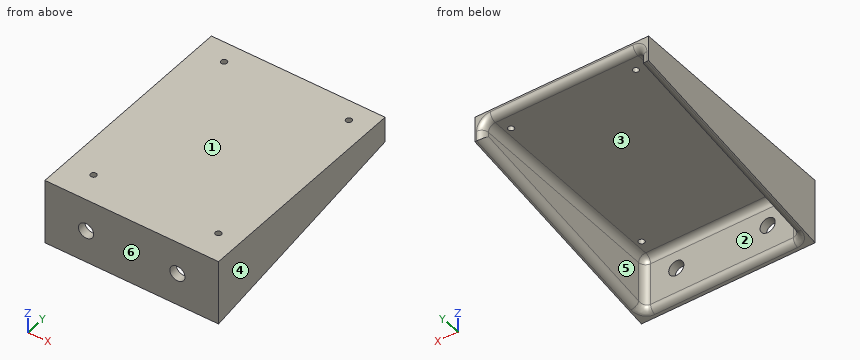
```python
from build123d import *

# Parameters (mm, degrees)
BOSS_EXTRUDE1_DEPTH        = 32.1564
SKETCH2_W                  = 57.9628
SKETCH2_H                  = 20.955
CUT_EXTRUDE1_DEPTH         = 80.772
M2_CLEARANCE_HOLE1_D       = 2.2
F_2_0_221_DIAMETER_HOLE1_D = 5.6134
FILLET1_R                  = 2.54


with BuildPart() as part:
    # Sketch1 → Boss-Extrude1 (new body, symmetric)
    with BuildSketch(Plane(origin=(0, 0, 0), x_dir=(0, 0, -1), z_dir=(1, 0, 0))):
        Polygon((0, 0), (24.13, 0), (9.4742, 83.947), (0, 83.947), align=None)
    extrude(amount=BOSS_EXTRUDE1_DEPTH, both=True)

    # Sketch2 → Cut-Extrude1 (cut)
    with BuildSketch(Plane(origin=(0, 83.947, 0), x_dir=(1, 0, 0), z_dir=(0, 1, 0))):
        with Locations((0, 13.6525)):
            Rectangle(SKETCH2_W, SKETCH2_H)
    extrude(amount=-CUT_EXTRUDE1_DEPTH, mode=Mode.SUBTRACT)

    # M2 Clearance Hole1 (through all)
    with Locations(Plane.XY):
        with Locations((-21.971, 76.454), (24.257, 76.454), (24.257, 10.668), (-21.971, 10.668)):
            Hole(M2_CLEARANCE_HOLE1_D / 2)

    # #2 (0.221) Diameter Hole1 (through all)
    with Locations(Plane(origin=(0, 0, 0), x_dir=(-1, 0, 0), z_dir=(0, -1, 0))):
        with Locations((-16.9164, 12.065), (16.9164, 12.065)):
            Hole(F_2_0_221_DIAMETER_HOLE1_D / 2)

    # Fillet1
    fillet1_edges = [part.edges().sort_by_distance(p)[0] for p in [
        (0, 3.175, -23.575695915),
        (28.9814, 43.561, -16.524947958),
        (-28.9814, 43.561, -16.524947958),
        (-28.9814, 43.561, -3.175),
        (-28.9814, 83.947, -6.3246),
        (0, 83.947, -3.175),
        (28.9814, 83.947, -6.3246),
        (28.9814, 3.175, -13.375347958),
        (0, 3.175, -3.175),
        (-28.9814, 3.175, -13.375347958),
        (28.9814, 43.561, -3.175),
    ]]
    fillet(fillet1_edges, radius=FILLET1_R)


solid = part.part
```
Part model, mm, in its own coordinate system. Face numbers are marked on the shaded views. A direction names the side the tool comes from. Coordinates: 2 decimals unless noted, no trailing zeros. Order: outer loops, then holes, each group sorted by start corner. A loop starts at its lowest first (then second) coordinate and runs counter-clockwise, first axis right, second up. Notation, with made-up numbers: (4.25, 86.5) -> (27.25, 86.5) arc R6 ccw to (27.25, 95.5) -> close; hole circle Ø10 at (36.5, 58). An arc over 180 degrees is marked (long way). Put each result on its own line as item: value. Start each with the question number.
(1) Band-saw the part on A-A (x = -7.5). Give the cut face in (y, z) (3 decimals).
(2) Probe line 1 along X through (y, z) = (8.5, -19.75); line 2 along Y through (x, z) = (-6.5, -8) (3 decimals); line 3 along Z through (x, y) = (23, 30) (3 decimals). List the from-to ranges inside material, lowest first. Write a range as [from, to].
(3) Pin check, flat tips, straight feed: pin 1 Ø4 at (x, y) = (-25.5, 17.5) entering from -Z; pin 2 Ø3.5 at (x, y) = (-21.971, 76.454) entering from -Z (3 decimals); pin 3 Ø6.5 at (x, z) = (16.92, -12.06) entering from +Y (3 decimals); pin 4 Ø1.3 at (x, y) = (24.257, 76.454) entering from -Z. Stop position of each tip, or through.
(4) Mould opens along X. For the marked faces 1, 2, 3 and 4 say: pulls with the +X half, pulls with the -X half, needs draft (parallel to the pull), parting line crosses it, or undercut.
(5) Which spindle directions (+Z, -Z, +X, -X, +Y, -Y) get a long thin tool onto all of the face, cutting with end or side? Do the marked faces 5 and 6. Say none if no direction does.
Determined:
1. outline: (0, -24.13) -> (1.072, -23.943) arc R2.54 ccw to (3.175, -21.441) -> (3.175, -5.715) arc R2.54 cw to (5.715, -3.175) -> (81.407, -3.175) arc R2.54 ccw to (83.947, -0.635) -> (83.947, 0) -> (0, 0) -> close
2. line 1: x = [-32.16, -28.98], [28.98, 32.16]
2. line 2: y = [0, 3.175]
2. line 3: z = [-3.175, 0]
3. pin 1: stops at z = -3.41
3. pin 2: stops at z = -3.175
3. pin 3: stops at y = 3.175
3. pin 4: passes through
4. face 1: needs draft
4. face 2: undercut
4. face 3: undercut
4. face 4: pulls with the +X half
5. face 5: -Z, +Y
5. face 6: +Z, -Z, +X, -X, -Y
